```python
from build123d import *

# Parameters (mm, degrees)
PAD_DEPTH         = 8.5
SKETCH003_R       = 109.254571
SKETCH003_R_2     = 59.25
POCKET_DEPTH      = 8.501
POCKET_DEPTH_BACK = -8.501


with BuildPart() as part:
    # Sketch → Pad (new body, symmetric)
    with BuildSketch(Plane.XY):
        with BuildLine():
            ThreePointArc((0, -37.5), (37.5, 0), (0, 37.5))
            Line((0, 37.5), (0, 5.8))
            Line((0, 5.8), (0, 5.1))
            Line((0, 3.4), (0, 5.1))
            Line((0, 3.4), (3.801316, 3.4))
            ThreePointArc((0, -5.1), (4.655642, -2.082066), (3.801316, 3.4))
            Line((0, -5.1), (0, -37.5))
        make_face()
    pad = extrude(amount=PAD_DEPTH, both=True)

    # Mirrored: Pad across Sketch V_Axis
    add(pad.mirror(Plane(origin=(0, 0, 0), x_dir=(0, 0, 1), z_dir=(1, 0, 0))))

    # Sketch001 → Groove (revolve, cut)
    with BuildSketch(Plane.YZ):
        Polygon((37.5, 0), (37.5, 5.6), (30.5, 2.6), (30.5, 0), align=None)
    groove = revolve(axis=Axis((0, 0, 0), (0, 0, 1)), mode=Mode.SUBTRACT)

    # Mirrored001: Groove across Sketch001 H_Axis
    add(groove.mirror(Plane.XY), mode=Mode.SUBTRACT)

    # Sketch003 → Pocket (cut, two sides)
    with BuildSketch(Plane.XY) as pocket_sk:
        Circle(SKETCH003_R)
        Circle(SKETCH003_R_2, mode=Mode.SUBTRACT)
    extrude(amount=-POCKET_DEPTH, mode=Mode.SUBTRACT)
    extrude(pocket_sk.sketch, amount=-POCKET_DEPTH_BACK, mode=Mode.SUBTRACT)


solid = part.part
```
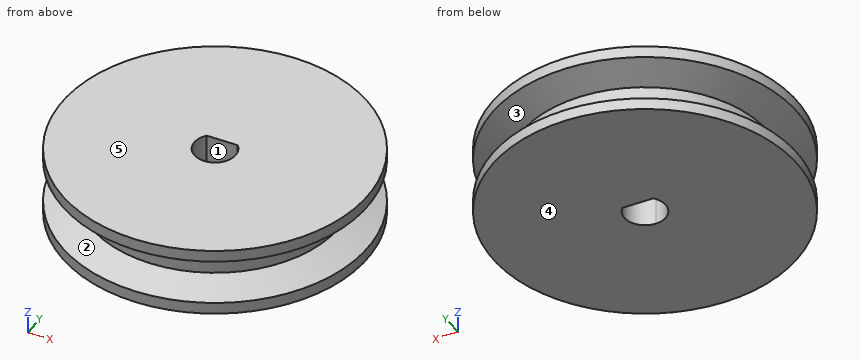
Can you work these out from the model? Positions are in its coordinate system, mm. Face numbers are marked on the shaded views. A direction names the side the tool comes from. Coordinates: 2 decimals unless noted, no trailing zeros. Loops run counter-clockwise (first coordinate to the right, second up) from the corner with the lowest first, then second, coordinate; pieces in that order, holes last.
1) Imagine slicing it at B-B on z = 6.5. List the corners of the cut face in (x, y) for me, plus the area to 3 significant figures.
2) Which directions (+Z, -Z, +X, -X, +Y, -Y) give clear straight access to the entire face, cutting with the end or side of a thin tool? Please do the marked faces 1 and 2.
3) Thinking about a two-plate mould opening in Z: for the marked faces 3, 4 and 5, which applies, pulls with the +Z half, pulls with the -Z half, needs draft (parallel to the pull), parting line crosses it, or undercut?
4) Imagine slicing it at A-A on y = 0. List the corners of the cut face in (x, z) for me, plus the area to 3 significant figures.
5) For pin 1 (3 mm diameter, centred on x = 13.5, z = -6.5, fed in from +Y); pin 2 (2.5 mm diameter, centred on x = -0.5, z = -1.5, fed in from -Y); pin 3 (10 mm diameter, centred on y = 28.5, z = 3, fed in from +X), each with a flat end and sliding along its axis, tell me the tip position at first contact or that it passes through.
6) I need wall thicknesses on probe 1 along Z at (x, y) = (31.5, 5); probe 2 along Z at (x, y) = (-18, -28.5); probe 3 along Y at (x, z) = (-4.5, 2.5). Which ranges of each line are inside material? Lowest first, please.
Completed:
1. outline: circle Ø75 at (0, 0); hole (-3.8, 3.4) arc R5.1 ccw (long way) to (3.8, 3.4) - close
1. area: 4,350 mm2
2. face 1: +Z, -Z
2. face 2: none
3. face 3: undercut
3. face 4: pulls with the -Z half
3. face 5: pulls with the +Z half
4. outline: (-37.5, -8.5) - (-5.1, -8.5) - (-5.1, 8.5) - (-37.5, 8.5) - (-37.5, 5.6) - (-30.5, 2.6) - (-30.5, -2.6) - (-37.5, -5.6) - close; (5.1, -8.5) - (37.5, -8.5) - (37.5, -5.6) - (30.5, -2.6) - (30.5, 2.6) - (37.5, 5.6) - (37.5, 8.5) - (5.1, 8.5) - close
4. area: 987 mm2
5. pin 1: stops at y = 35.53
5. pin 2: stops at y = -30.85
5. pin 3: stops at x = 28.62
6. probe 1: z = -8.5 to -3.2, 3.2 to 8.5
6. probe 2: z = -8.5 to -3.97, 3.97 to 8.5
6. probe 3: y = -30.17 to -2.4, 2.4 to 30.17
